Can you work these out from the model? Positions are in its coordinate system, mm. A direction names the side the tool comes from. Coordinates: 2 decimals unless noted, no trailing zeros. Write each loop counter-clockwise with the first axis right and the second up, starting at its lowest first coordinate (ties: lowest second). Pieces come first, ordered by that corner, then holes. Notation, with made-up numbers: (-1.75, 13) - (31.25, 13) arc R18 cw to (31.25, 21) - close; hole circle Ø11 at (12, 83.25). An arc over 180 degrees is marked (long way). Write each question's results on one line, items separated by ' | '. Start each with the question number.
```python
from build123d import *

# Parameters (mm, degrees)
SKETCH1_R            = 15.75
SKETCH1_R_2          = 12.75
BOSS_EXTRUDE1_DEPTH  = 5
FILLET3_R            = 1
SKETCH1_3_R          = 12.75
SKETCH1_3_R_2        = 11.5
BOSS_EXTRUDE29_DEPTH = 1


with BuildPart() as part:
    # Sketch1 → Boss-Extrude1 (new body)
    with BuildSketch(Plane(origin=(0, 0, 0), x_dir=(0, 0, -1), z_dir=(1, 0, 0))):
        Circle(SKETCH1_R)
        Circle(SKETCH1_R_2, mode=Mode.SUBTRACT)
    extrude(amount=-BOSS_EXTRUDE1_DEPTH)

    # Fillet3
    fillet3_edges = [part.edges().sort_by_distance(p)[0] for p in [
        (-5, 0, 12.75),
    ]]
    fillet(fillet3_edges, radius=FILLET3_R)

    # Sketch1<3> → Boss-Extrude29 (add)
    with BuildSketch(Plane(origin=(0, 0, 0), x_dir=(0, 0, -1), z_dir=(1, 0, 0))):
        Circle(SKETCH1_3_R)
        Circle(SKETCH1_3_R_2, mode=Mode.SUBTRACT)
    extrude(amount=-BOSS_EXTRUDE29_DEPTH)


solid = part.part
```
Q1. I need wall thicknesses on line 1 along Y through (x, z) = (-0.4, 0); line 2 along Y through (x, z) = (-1.7, 0); line 3 along Z through (x, y) = (-2.85, 10). Which ranges of each line are inside material? Lowest first, please. Write a range as from..to.
Q2. If we section it at A-A (z = 0): Please give me the cut outline in (x, y).
Q3. Thinking about a two-plate mould opening in Y: for faces 3 (the face through (-2.465, 15.616, 2.05)), 4 (the face through (0, -12, -1)), 5 (the face through (-2.479, -12.447, 2.764)), which applies, pulls with the +Y half, pulls with the -Y half, needs draft (parallel to the pull), parting line crosses it, or undercut?
Q4. For faces 1 (the face through (-5, -14, 0)), 2 (the face through (-1, 10, 7)), which set-ups out of +Z, -Z, +X, -X, +Y, -Y let a thin tool reach every point of the face, with its end or its side?
Q5. I'm going to push flat-ended pins straight in: pin 1 Ø2 at (x, z) = (-4.5, 0.5) entering from -Y; pin 2 Ø2 at (x, z) = (-2, -4.5) entering from +Y. Where does each tip first touch, or does it pass through?
Q6. If we section it at C-C (x = -3.3): Please give me the cut outline in (y, z).
Answer list:
1) line 1: y = -15.75..-11.5, 11.5..15.75 | line 2: y = -15.75..-12.75, 12.75..15.75 | line 3: z = -12.17..-7.91, 7.91..12.17
2) outline: (-5, -15.75) - (0, -15.75) - (0, -11.5) - (-1, -11.5) - (-1, -12.75) - (-4, -12.75) arc R1 ccw to (-5, -13.75) - close; (-5, 13.75) arc R1 ccw to (-4, 12.75) - (-1, 12.75) - (-1, 11.5) - (0, 11.5) - (0, 15.75) - (-5, 15.75) - close
3) face 3: parting line crosses it | face 4: needs draft | face 5: undercut
4) face 1: +Z, -Z, -X, +Y, -Y | face 2: -X
5) pin 1: stops at y = -15.75 | pin 2: stops at y = 15.36
6) outline: circle Ø31.5 at (0, 0); hole circle Ø25.5 at (0, 0)
